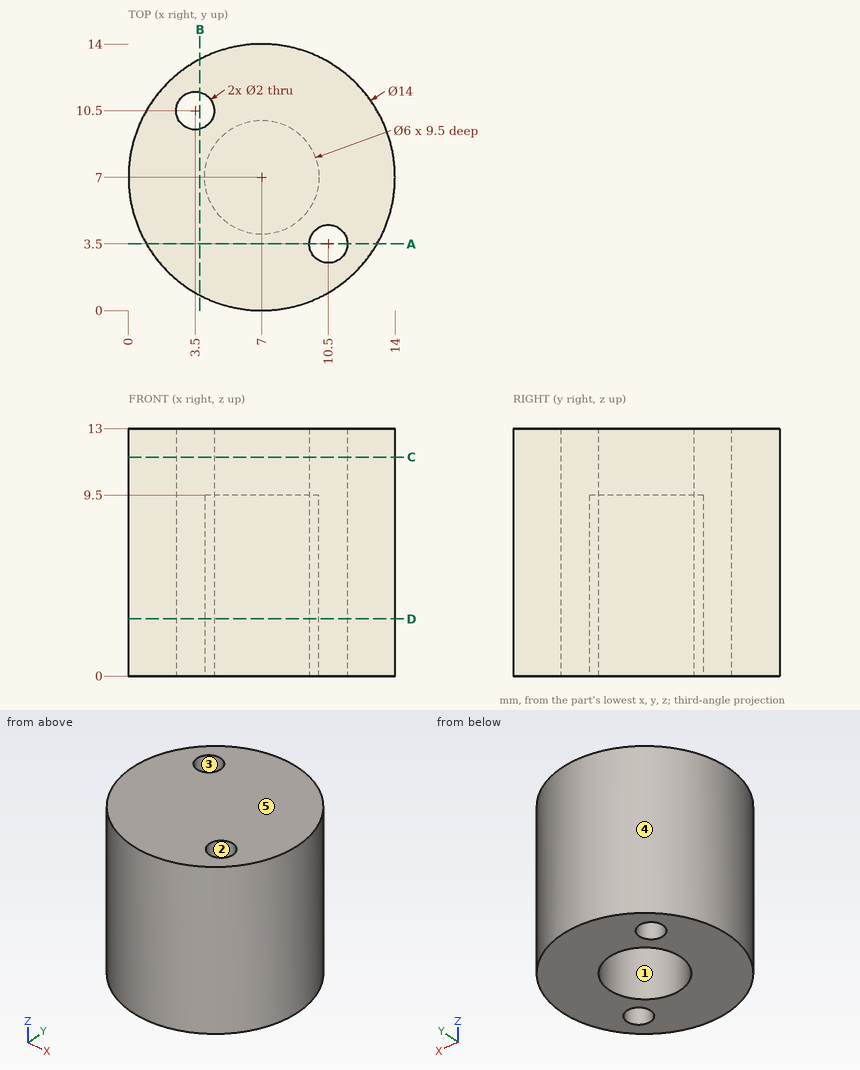
Study the drawing (mm; zero at the part's minimum x, y, z) and answer. A direction names the side the tool comes from. Give positions to 0.01 mm unless a question says otherwise; leave off trailing zeros. Write each loop counter-clockwise with the first axis right and the second up, starting at its lowest first coordinate (ties: lowest second). Pieces come first, ordered by that corner, then holes.
(1) The part is cut by section D-D on z = 3. Write down the section's boundary in (x, y).
Final values:
outline: circle Ø14 at (7, 7); hole circle Ø2 at (3.5, 10.5); hole circle Ø6 at (7, 7); hole circle Ø2 at (10.5, 3.5)
(2) The part is cut by section C-C on z = 11.5. Write down the section's boundary in (x, y), plus the area to 3 significant figures.
Final values:
outline: circle Ø14 at (7, 7); hole circle Ø2 at (3.5, 10.5); hole circle Ø2 at (10.5, 3.5)
area: 148 mm2
(3) The part is cut by section A-A on y = 3.5. Write down the section's boundary in (x, z).
Final values:
outline: (0.94, 0) - (9.5, 0) - (9.5, 13) - (0.94, 13) - close; (11.5, 0) - (13.06, 0) - (13.06, 13) - (11.5, 13) - close
(4) Flat-ended cylindrical pins translate along their axes: pin 1 Ø1.5 at (x, z) = (11.5, 11.5) entering from +Y; pin 2 Ø1.8 at (x, y) = (7.5, 8) entering from -Z; pin 3 Ø5 at (y, z) = (11.5, 3) entering from -X. Find the tip coordinate at first contact, or state that the pin passes through.
Final values:
pin 1: stops at y = 12.91
pin 2: stops at z = 9.5
pin 3: stops at x = 0.29
(5) Which of the six approach directions +Z, -Z, +X, -X, +Y, -Y give full straight-line access (tool end or side, diameter ignored) to the marked faces 1 and 2?
Final values:
face 1: -Z
face 2: +Z, -Z
(6) The mould has two halves that part along Y. Classify the marked faces 3, 4 and 5: pulls with the +Y half, pulls with the -Y half, needs draft (parallel to the pull), parting line crosses it, or undercut.
Final values:
face 3: undercut
face 4: parting line crosses it
face 5: needs draft
(7) The part is cut by section B-B on x = 3.75. Write down the section's boundary in (y, z), plus the area to 3 significant figures.
Final values:
outline: (0.8, 0) - (9.53, 0) - (9.53, 13) - (0.8, 13) - close; (11.47, 0) - (13.2, 0) - (13.2, 13) - (11.47, 13) - close
area: 136 mm2
(8) Straight lines are drawn through the part: line 1 (Y direction, x = 7, z = 7.75); line 2 (Y direction, x = 3, z = 11); line 3 (X direction, y = 3.5, z = 3). For each, find the intervals that lie inside material, in ascending order.
Final values:
line 1: y = 0 to 4, 10 to 14
line 2: y = 1.26 to 9.63, 11.37 to 12.74
line 3: x = 0.94 to 9.5, 11.5 to 13.06
